For this review, take the finished solid that the model builds, in its own axes (mm). A direction names the side the tool comes from. Round coordinates to 2 decimals unless told otherwise and drop trailing zeros. Order: outer loops, then holes, each group sorted by start corner. A loop starts at its lowest first (then second) coordinate and runs counter-clockwise, first axis right, second up. Notation, with made-up numbers: M 86.5,-16 L 138.5,-16 A11 ccw 138.5,-8 Z; hole C -31.5,40 d3. An arc over 180 degrees is marked long. Answer as a JSON object with one key per item and string values.
from build123d import *

# Parameters (mm, degrees)
BASE_SKETCH_W           = 42
BASE_SKETCH_H           = 20
BASE_DEPTH              = 10
MOUNT_SCREW_D           = 6.6
MOUNT_SCREW_CBORE_D     = 11
MOUNT_SCREW_CBORE_DEPTH = 6.4
PROFILE_CLIP_DEPTH      = 3
ZAOBLIT1_R              = 5


with BuildPart() as part:
    # Base sketch → Base (new body)
    with BuildSketch(Plane.XY):
        Rectangle(BASE_SKETCH_W, BASE_SKETCH_H)
    extrude(amount=BASE_DEPTH)

    # Mount screw (through all)
    with Locations(Plane.XY.offset(10)):
        with Locations((0, 0)):
            CounterBoreHole(MOUNT_SCREW_D / 2, MOUNT_SCREW_CBORE_D / 2, MOUNT_SCREW_CBORE_DEPTH)

    # Profile clip sketch → Profile clip (add)
    with BuildSketch(Plane(origin=(0, 0, 0), x_dir=(-1, 0, 0), z_dir=(0, 0, -1))):
        with BuildLine():
            Line((-8.062257748, 4), (-21, 4))
            Line((-21, 4), (-21, -4))
            Line((-21, -4), (-8.062257748, -4))
            ThreePointArc((-8.062257748, -4), (-9, 0), (-8.062257748, 4))
        make_face()
        with BuildLine():
            Line((21, 4), (8.062257748, 4))
            ThreePointArc((8.062257748, 4), (8.762428879, 2.054224947), (9, 0))
            ThreePointArc((9, 0), (8.762428879, -2.054224947), (8.062257748, -4))
            Line((8.062257748, -4), (21, -4))
            Line((21, -4), (21, 4))
        make_face()
    extrude(amount=PROFILE_CLIP_DEPTH)

    # Zaoblit1
    zaoblit1_edges = [part.edges().sort_by_distance(p)[0] for p in [
        (21, -10, 5),
        (-21, -10, 5),
        (-21, 10, 5),
        (21, 10, 5),
    ]]
    fillet(zaoblit1_edges, radius=ZAOBLIT1_R)


solid = part.part
1) Add section A-A on z = -2. State the section outline as (x, y) points.
Geometry check:
{"outline": "M -21,-4 L -8.06,-4 A9 cw -8.06,4 L -21,4 Z; M 8.06,-4 L 21,-4 L 21,4 L 8.06,4 A9 cw Z"}
2) Add section B-B on x = -12.5. State the section outline as (y, z) points, and give its area (3 significant figures).
Geometry check:
{"outline": "M -10,0 L -4,0 L -4,-3 L 4,-3 L 4,0 L 10,0 L 10,10 L -10,10 Z", "area": "224 mm²"}
3) Add section C-C on y = -0.5. State the section outline as (x, z) points.
Geometry check:
{"outline": "M -21,-3 L -8.99,-3 L -8.99,0 L -3.26,0 L -3.26,3.6 L -5.48,3.6 L -5.48,10 L -21,10 Z; M 3.26,0 L 8.99,0 L 8.99,-3 L 21,-3 L 21,10 L 5.48,10 L 5.48,3.6 L 3.26,3.6 Z"}
4) Insertion check: P1, Ø1.5, axis at x = -16.5, z = -1, coming from the -Y side; P2, Ø7.5, axis at x = 0, y = 0, coming from the -Z side. Each pin has a flat end and moves straight along its axis. Give the tip position at first contact, or say it passes through.
Geometry check:
{"P1": "stops at y = -4", "P2": "stops at z = 0"}
5) Add section D-D on x = 0. State the section outline as (y, z) points, and give its area (3 significant figures).
Geometry check:
{"outline": "M -10,0 L -3.3,0 L -3.3,3.6 L -5.5,3.6 L -5.5,10 L -10,10 Z; M 3.3,0 L 10,0 L 10,10 L 5.5,10 L 5.5,3.6 L 3.3,3.6 Z", "area": "106 mm²"}
6) Machinability: for faces 4 (the flat face through (4, 0, 3.6)), 5 (the flat face through (14, 4, -1)), 6 (the cylindrical face through (9, 0, -1)), 7 (the flat face through (-14, -4, -1)), which of the approach directions +Z, -Z, +X, -X, +Y, -Y give a long, thin tool a straight path to every point of the face, cutting with its end or side? Answer none if there is none.
Geometry check:
{"face 4": "+Z", "face 5": "-Z, +X, -X, +Y", "face 6": "-Z", "face 7": "-Z, +X, -X, -Y"}
7) Mouldability with a two-part tool opening along X and no side actions: class faces 1 (the flat face through (0, -10, 5)), 2 (the flat face through (-21, 0, 3)), 3 (the cylindrical face through (-1.19, -5.37, 6.84)) as +X half, -X half, draft (parallel to the pull), parting line (faces both ways), or undercut.
Geometry check:
{"face 1": "draft", "face 2": "-X half", "face 3": "undercut"}
8) For L1, parallel to Y at x = 0, z = 8.5; L2, parallel to Y at x = 0, z = 1; L3, parallel to Z at x = -5.5, y = 9, list the stretches that pass through material, from the lowest coordinate up.
Geometry check:
{"L1": "y = -10 to -5.5, 5.5 to 10", "L2": "y = -10 to -3.3, 3.3 to 10", "L3": "z = 0 to 10"}
